Check sheet for the modelled part. Datum: model origin and axes. Units: mm. A direction names the side the tool comes from. Coordinates: 2 decimals unless noted, no trailing zeros. Loops run counter-clockwise (first coordinate to the right, second up) from the corner with the lowest first, then second, coordinate; pieces in that order, holes last. Notation, with made-up numbers: M 9,-17 L 63,-17 A23 ccw 63,0 Z; hole C 72,64.25 d8. An arc over 180 degrees is marked long. Use CSV: the item, a comma, the result in double quotes. Start each with the question number.
(1) Section check B-B on z = -20.25. Record the cut outline in (x, y), and give its area (3 significant figures).
(2) Section check A-A on y = 6. Record the cut outline in (x, z) (3 decimals), and give its area (3 significant figures).
(3) Draft check along Z on faces 1 (the flat face through (-88, 4, -5.781)), 2 (the flat face through (-29.546, 4, -10)), 3 (the flat face through (-37, 2, -23)). Enter one of: pulls with the +Z half, pulls with the -Z half, needs draft (parallel to the pull), parting line crosses it, or undercut.
(4) Scan lines: line 1 (Z direction, x = -141.5, y = 4.5); line 2 (X direction, y = 2.5, z = -8.75); line 3 (Z direction, x = -40.5, y = 1.25). Record each from-to range of solid material in increasing order.
(5) Set-up check for faces 4 (the flat face through (-34, 1, -16.206)), 5 (the flat face through (-34, 5, -24.781)), 6 (the flat face through (-143, 5, -24.781)), 7 (the flat face through (-143, 1, -22.356)): record each of +Z, -Z, +X, -X, +Y, -Y from which the full face is reachable in a straight line by a thin tool's end or side.
(6) Go/stop test with flat-tipped pins: pin 1 Ø1.5 at (y, z) = (4, -16) entering from -X; pin 2 Ø1 at (y, z) = (6, -17) entering from +X. Record where each tip stops, or that it passes through.
Autodesk Inventor part; units mm, degrees
ref_plane "YZ Plane" through (0, 0, 0) normal (1, 0, 0) x (0, 1, 0)
ref_plane "XZ Plane" through (0, 0, 0) normal (0, 1, 0) x (-1, 0, 0)
ref_plane "XY Plane" through (0, 0, 0) normal (0, 0, 1) x (1, 0, 0)
sketch "Sketch1" plane through (0, 0, 0) normal (0, 1, 0) x (-1, 0, 0)
  circle A0 centre (118.5461, -28.7809) radius 1.975
  circle A1 centre (118.5461, -9.7809) radius 1.49
  arc A2 (138.5461, -13.7809) -> (138.5461, -24.7809) centre (138.5461, -19.2809) ccw
  circle A3 centre (58.5461, -28.8073) radius 1.975
  line L0 (147.5461, -32.7809) -> (29.5461, -32.7809)
  line L1 (29.5461, -5.7809) -> (147.5461, -5.7809)
  arc A4 (38.5461, -24.7809) -> (38.5461, -13.7809) centre (38.5461, -19.2809) ccw
  line L2 (29.5461, -32.7809) -> (29.5461, -5.7809)
  circle A5 centre (58.5461, -9.8073) radius 1.49
  arc A6 (138.5461, -16.2059) -> (138.5461, -22.3559) centre (138.5461, -19.2809) ccw
  arc A7 (38.5461, -22.3559) -> (38.5461, -16.2059) centre (38.5461, -19.2809) ccw
  line L3 (143.1062, -22.3559) -> (147.5461, -22.3559)
  line L4 (143.1062, -16.2059) -> (147.5461, -16.2059)
  line L5 (147.5461, -32.7809) -> (147.5461, -22.3559)
  line L6 (147.5461, -16.2059) -> (147.5461, -5.7809)
  line L7 (143.1062, -22.3559) -> (138.5461, -22.3559)
  line L8 (143.1062, -16.2059) -> (138.5461, -16.2059)
  line L9 (138.5461, -24.7809) -> (147.5461, -24.7809)
  line L10 (138.5461, -13.7809) -> (147.5461, -13.7809)
  line L11 (38.5461, -22.3559) -> (29.5461, -22.3559)
  line L12 (38.5461, -24.7809) -> (29.5461, -24.7809)
  line L13 (38.5461, -16.2059) -> (29.5461, -16.2059)
  line L14 (38.5461, -13.7809) -> (29.5461, -13.7809)
  point P0 (88.5461, -32.7809)
  point P1 (88.5461, -5.7809)
  dimension "d162" = 60
  dimension "d163" = 60
  dimension "d165" = 100
  dimension "d183" = 11
  dimension "d184" = 11
  dimension "d185" = 6.15
  dimension "d186" = 6.15
  dimension "d187" = 3.95
  dimension "d188" = 2.98
  dimension "d189" = 3.95
  dimension "d190" = 2.98
  dimension "d202" = 9
  dimension "d203" = 9
  dimension "d204" = 9
  dimension "d212" = 19
  dimension "d213" = 19
  dimension "d214" = 27
  dimension "d215" = 4
  dimension "d216" = 4
  dimension "d217" = 13.5
  dimension "d218" = 30
  dimension "d219" = 30
extrude "Extrusion13" add sketch "Sketch1" along normal blind 8 contours A2 L9 L5 L0 L2 L12 A4 L14 L1 L6 L10
extrude "Extrusion14" add sketch "Sketch1" along normal blind 2 contours L14 A4 L12 L2 L11 A7 L13
extrude "Extrusion15" add sketch "Sketch1" along normal blind 2 contours L10 L6 L4 L8 A6 L7 L3 L5 L9 A2
properties part number "Base Laser_3DPrint"
Outcome:
1,outline,"M -135.63,0 L -41.46,0 L -41.46,2 L -43.96,2 L -43.96,8 L -133.13,8 L -133.13,2 L -135.63,2 Z"
1,area,"723 mm²"
2,outline,"M -147.546,-32.781 L -29.546,-32.781 L -29.546,-24.781 L -38.546,-24.781 A5.5 cw -38.546,-13.781 L -29.546,-13.781 L -29.546,-5.781 L -147.546,-5.781 L -147.546,-13.781 L -138.546,-13.781 A5.5 cw -138.546,-24.781 L -147.546,-24.781 Z; hole C -118.546,-28.781 d3.95; hole C -118.546,-9.781 d2.98; hole C -58.546,-28.807 d3.95; hole C -58.546,-9.807 d2.98"
2,area,"2,850 mm²"
3,face 1,"pulls with the +Z half"
3,face 2,"needs draft"
3,face 3,"undercut"
4,line 1,"z = -32.78 to -24.78, -13.78 to -5.78"
4,line 2,"x = -147.55 to -119.62, -117.47 to -59.6, -57.5 to -29.55"
4,line 3,"z = -32.78 to -21.66, -16.91 to -5.78"
5,face 4,"+X, +Y, -Y"
5,face 5,"+X, +Y"
5,face 6,"-X, +Y"
5,face 7,"-X, +Y, -Y"
6,pin 1,"stops at x = -134.8"
6,pin 2,"stops at x = -43.29"
